Verification items for the finished model (mm, model axes). A direction names the side the tool comes from. Coordinates: 2 decimals unless noted, no trailing zeros. Loops run counter-clockwise (first coordinate to the right, second up) from the corner with the lowest first, then second, coordinate; pieces in that order, holes last. Notation, with made-up numbers: (80.25, 10) - (86.25, 10) arc R28 ccw to (86.25, 44) - close; hole circle Ø8 at (-3, -27). An arc over 180 degrees is marked (long way). Answer as CSV lines item,"result". Start each with the question number.
1. Material ranges on line 1 (X direction, y = -1.5, z = 14); line 2 (Z direction, x = 40.8, y = -11.3); line 3 (Y direction, x = 81.6, z = 13.5), recorded low to high. Write a range as [from, to].
2. Cross-section at D-D (z = 26). Enter the section's corners in (x, y), plus the area to 3 significant figures.
3. Set-up check for faces 1 (the cylindrical face through (70.21, 3.78, 34.17)), 2 (the flat face through (74.84, 6.99, 34.17)), 3 (the flat face through (21.503, 15.216, 5.677)), 4 (the cylindrical face through (60.177, 15.018, 0.143)), 5 (the cylindrical face through (39.759, -11.392, 27.932)): record each of +Z, -Z, +X, -X, +Y, -Y from which the full face is reachable in a straight line by a thin tool's end or side.
4. Cross-section at A-A (z = 20). Enter the section's corners in (x, y).
5. Gauge pin test, flat ends, axial feed: P1, Ø5, axis at x = 35.3, y = 17.5, coming from the +Z side; P2, Ø14.5, axis at x = 40.8, z = 45, coming from the +Y side; P3, Ø4, axis at y = -3.5, z = 41, coming from the +X side. Record the tip position at first contact, or that the pin passes through.
6. Release check for a two-part mould opening along Z. For faces 6 (the cylindrical face through (-7.493, 0.33, 28.594)), 7 (the cylindrical face through (21.423, 15.018, 0.143)), 8 (the cylindrical face through (39.759, -11.392, 52.932)) record: pulls with the +Z half, pulls with the -Z half, needs draft (parallel to the pull), parting line crosses it, or undercut.
7. Cross-section at B-B (x = 39). State how many separate pieces and enclosed holes the cut face has, plus the area to 3 significant figures.
8. Cross-section at C-C (z = 33). Enter the section's corners in (x, y), plus the area to 3 significant figures.
```python
from build123d import *

# Parameters (mm, degrees)
CYLINDER010_R          = 3.2
CYLINDER010_DEPTH      = 40
CYLINDER011_R          = 3.2
CYLINDER011_DEPTH      = 40
CYLINDER012_R          = 8
CYLINDER012_DEPTH      = 1.2
CYLINDER013_R          = 8
CYLINDER013_DEPTH      = 1.2
BOX002_W               = 2
BOX002_H               = 10
BOX002_DEPTH           = 60
BOX002_PLACEMENT_ANGLE = 45
BOX003_W               = 2
BOX003_H               = 10
BOX003_DEPTH           = 60
BOX003_PLACEMENT_ANGLE = 45
CYLINDER006_R          = 2
CYLINDER006_DEPTH      = 20
CYLINDER007_R          = 2
CYLINDER007_DEPTH      = 20
CYLINDER008_R          = 2
CYLINDER008_DEPTH      = 20
CYLINDER009_R          = 2
CYLINDER009_DEPTH      = 20
CYLINDER005_R          = 12
CYLINDER005_DEPTH      = 4
CYLINDER004_R          = 5.5
CYLINDER004_DEPTH      = 20
CYLINDER002_R          = 7.5
CYLINDER002_DEPTH      = 58
CYLINDER_R             = 7.5
CYLINDER_DEPTH         = 58
BOX001_W               = 81.6
BOX001_H               = 33
BOX001_DEPTH           = 11
CHAMFER_1_SIZE2        = 35
CHAMFER_1_SIZE         = 15
CHAMFER_2_SIZE2        = 35
CHAMFER_2_SIZE         = 15
CYLINDER001_R          = 12
CYLINDER001_DEPTH      = 58
CYLINDER003_R          = 12
CYLINDER003_DEPTH      = 58
BOX_W                  = 81.6
BOX_H                  = 12
BOX_DEPTH              = 58
FILLET_R               = 0.5


with BuildPart() as cylinder:
    # Cylinder010 → Cylinder010 (new body)
    with BuildSketch(Plane(origin=(40.8, 20, 20), x_dir=(1, 0, 0), z_dir=(0, -1, 0))):
        Circle(CYLINDER010_R)
    extrude(amount=CYLINDER010_DEPTH)


with BuildPart() as cylinder001:
    # Cylinder011 → Cylinder011 (new body)
    with BuildSketch(Plane(origin=(40.8, 20, 45), x_dir=(1, 0, 0), z_dir=(0, -1, 0))):
        Circle(CYLINDER011_R)
    extrude(amount=CYLINDER011_DEPTH)


with BuildPart() as cylinder002:
    # Cylinder012 → Cylinder012 (new body)
    with BuildSketch(Plane(origin=(40.8, -10.8, 20), x_dir=(1, 0, 0), z_dir=(0, -1, 0))):
        Circle(CYLINDER012_R)
    extrude(amount=CYLINDER012_DEPTH)


with BuildPart() as cylinder003:
    # Cylinder013 → Cylinder013 (new body)
    with BuildSketch(Plane(origin=(40.8, -10.8, 45), x_dir=(1, 0, 0), z_dir=(0, -1, 0))):
        Circle(CYLINDER013_R)
    extrude(amount=CYLINDER013_DEPTH)


with BuildPart() as obj1:
    # Box002 → Box002 (new body)
    with BuildSketch(Plane.XY):
        with Locations((1, 5)):
            Rectangle(BOX002_W, BOX002_H)
    extrude(amount=BOX002_DEPTH)


with BuildPart() as obj1_1:
    # Box002 placement: moved
    add(obj1.part.moved(Location((77, 2, 11))).rotate(Axis((77, 2, 11), (0, 0, 1)), BOX002_PLACEMENT_ANGLE))


with BuildPart() as obj2:
    # Box003 → Box003 (new body)
    with BuildSketch(Plane.XY):
        with Locations((1, 5)):
            Rectangle(BOX003_W, BOX003_H)
    extrude(amount=BOX003_DEPTH)


with BuildPart() as obj2_1:
    # Box003 placement: moved
    add(obj2.part.moved(Location((3, 3, 11))).rotate(Axis((3, 3, 11), (0, 0, -1)), BOX003_PLACEMENT_ANGLE))


with BuildPart() as zylinder006:
    # Cylinder006 → Cylinder006 (new body)
    with BuildSketch(Plane(origin=(35.3, 6.5, 0), x_dir=(1, 0, 0), z_dir=(0, 0, 1))):
        Circle(CYLINDER006_R)
    extrude(amount=CYLINDER006_DEPTH)


with BuildPart() as zylinder007:
    # Cylinder007 → Cylinder007 (new body)
    with BuildSketch(Plane(origin=(35.3, 17.5, 0), x_dir=(1, 0, 0), z_dir=(0, 0, 1))):
        Circle(CYLINDER007_R)
    extrude(amount=CYLINDER007_DEPTH)


with BuildPart() as zylinder008:
    # Cylinder008 → Cylinder008 (new body)
    with BuildSketch(Plane(origin=(46.3, 6.5, 0), x_dir=(1, 0, 0), z_dir=(0, 0, 1))):
        Circle(CYLINDER008_R)
    extrude(amount=CYLINDER008_DEPTH)


with BuildPart() as zylinder009:
    # Cylinder009 → Cylinder009 (new body)
    with BuildSketch(Plane(origin=(46.3, 17.5, 0), x_dir=(1, 0, 0), z_dir=(0, 0, 1))):
        Circle(CYLINDER009_R)
    extrude(amount=CYLINDER009_DEPTH)


with BuildPart() as zylinder005:
    # Cylinder005 → Cylinder005 (new body)
    with BuildSketch(Plane(origin=(40.8, 12, 7), x_dir=(1, 0, 0), z_dir=(0, 0, 1))):
        Circle(CYLINDER005_R)
    extrude(amount=CYLINDER005_DEPTH)


with BuildPart() as zylinder004:
    # Cylinder004 → Cylinder004 (new body)
    with BuildSketch(Plane(origin=(40.8, 12, 0), x_dir=(1, 0, 0), z_dir=(0, 0, 1))):
        Circle(CYLINDER004_R)
    extrude(amount=CYLINDER004_DEPTH)


with BuildPart() as zylinder002:
    # Cylinder002 → Cylinder002 (new body)
    with BuildSketch(Plane(origin=(81.6, 0, 0), x_dir=(1, 0, 0), z_dir=(0, 0, 1))):
        Circle(CYLINDER002_R)
    extrude(amount=CYLINDER002_DEPTH)


with BuildPart() as zylinder:
    # Cylinder → Cylinder (new body)
    with BuildSketch(Plane.XY):
        Circle(CYLINDER_R)
    extrude(amount=CYLINDER_DEPTH)


with BuildPart() as chamfer_body:
    # Box001 → Box001 (new body)
    with BuildSketch(Plane(origin=(0, -12, 0), x_dir=(1, 0, 0), z_dir=(0, 0, 1))):
        with Locations((40.8, 16.5)):
            Rectangle(BOX001_W, BOX001_H)
    extrude(amount=BOX001_DEPTH)

    # Chamfer 1
    chamfer_1_edges = [chamfer_body.edges().sort_by_distance(p)[0] for p in [
        (81.6, 21, 5.5),
    ]]
    chamfer_1_side = chamfer_body.faces().sort_by_distance((81.6, 4.5, 5.5))[0]
    chamfer(chamfer_1_edges, length=CHAMFER_1_SIZE, length2=CHAMFER_1_SIZE2, reference=chamfer_1_side)

    # Chamfer 2
    chamfer_2_edges = [chamfer_body.edges().sort_by_distance(p)[0] for p in [
        (0, 21, 5.5),
    ]]
    chamfer_2_side = chamfer_body.faces().sort_by_distance((0, 4.5, 5.5))[0]
    chamfer(chamfer_2_edges, length=CHAMFER_2_SIZE, length2=CHAMFER_2_SIZE2, reference=chamfer_2_side)


with BuildPart() as zylinder001:
    # Cylinder001 → Cylinder001 (new body)
    with BuildSketch(Plane.XY):
        Circle(CYLINDER001_R)
    extrude(amount=CYLINDER001_DEPTH)


with BuildPart() as zylinder003:
    # Cylinder003 → Cylinder003 (new body)
    with BuildSketch(Plane(origin=(81.6, 0, 0), x_dir=(1, 0, 0), z_dir=(0, 0, 1))):
        Circle(CYLINDER003_R)
    extrude(amount=CYLINDER003_DEPTH)


with BuildPart() as fillet_body:
    # Box → Box (new body)
    with BuildSketch(Plane(origin=(0, -12, 0), x_dir=(1, 0, 0), z_dir=(0, 0, 1))):
        with Locations((40.8, 6)):
            Rectangle(BOX_W, BOX_H)
    extrude(amount=BOX_DEPTH)

    # Fusion: union Chamfer body, Zylinder001, Zylinder003
    add(chamfer_body.part)
    add(zylinder001.part)
    add(zylinder003.part)

    # Cut: cut Zylinder
    add(zylinder.part, mode=Mode.SUBTRACT)

    # Cut001: cut Zylinder002
    add(zylinder002.part, mode=Mode.SUBTRACT)

    # Cut002: cut Zylinder004
    add(zylinder004.part, mode=Mode.SUBTRACT)

    # Cut003: cut Zylinder005
    add(zylinder005.part, mode=Mode.SUBTRACT)

    # Cut004: cut Zylinder009
    add(zylinder009.part, mode=Mode.SUBTRACT)

    # Cut005: cut Zylinder008
    add(zylinder008.part, mode=Mode.SUBTRACT)

    # Cut006: cut Zylinder007
    add(zylinder007.part, mode=Mode.SUBTRACT)

    # Cut007: cut Zylinder006
    add(zylinder006.part, mode=Mode.SUBTRACT)

    # Cut008: cut obj2
    add(obj2_1.part, mode=Mode.SUBTRACT)

    # Cut009: cut obj1
    add(obj1_1.part, mode=Mode.SUBTRACT)

    # Cut010: cut Cylinder003
    add(cylinder003.part, mode=Mode.SUBTRACT)

    # Cut011: cut Cylinder002
    add(cylinder002.part, mode=Mode.SUBTRACT)

    # Cut012: cut Cylinder001
    add(cylinder001.part, mode=Mode.SUBTRACT)

    # Cut013: cut Cylinder
    add(cylinder.part, mode=Mode.SUBTRACT)

    # Fillet
    fillet_edges = [fillet_body.edges().sort_by_distance(p)[0] for p in [
        (-11.296167, 4.049272, 0),
        (40.8, -12, 0),
        (21.311771, 15.133616, 0),
        (40.8, 21, 0),
        (60.288229, 15.133616, 0),
        (86.724329, 10.850864, 0),
        (90.085281, -8.485281, 0),
    ]]
    fillet(fillet_edges, radius=FILLET_R)


solid = fillet_body.part
```
Values follow:
1,line 1,"x = [-11.91, -7.35], [7.35, 74.25], [88.95, 93.51]"
1,line 2,"z = [0, 12], [28, 37], [53, 58]"
1,line 3,"y = [-12, -7.5], [7.5, 12]"
2,outline,"(0, -12) - (35.51, -12) - (35.51, -10.8) - (46.09, -10.8) - (46.09, -12) - (81.6, -12) arc R12 ccw (long way) to (73.23, 8.6) - (76.41, 5.42) arc R7.5 cw (long way) to (75.16, 3.84) - (71.91, 7.09) arc R12 ccw to (69.6, 0) - (12, 0) arc R12 ccw to (9.78, 6.95) - (6.53, 3.7) arc R7.5 cw (long way) to (5.3, 5.3) - (8.49, 8.49) arc R12 ccw (long way) to start"
2,area,"1,270 mm²"
3,face 1,"+Z, +Y"
3,face 2,"+Z"
3,face 3,"+Z, -Z, +Y"
3,face 4,"-Z, +Y"
3,face 5,"-Y"
4,outline,"(0, -12) - (32.8, -12) - (32.8, -10.8) - (37.6, -10.8) - (37.6, 0) - (12, 0) arc R12 ccw to (9.78, 6.95) - (6.53, 3.7) arc R7.5 cw (long way) to (5.3, 5.3) - (8.49, 8.49) arc R12 ccw (long way) to start; (44, -10.8) - (48.8, -10.8) - (48.8, -12) - (81.6, -12) arc R12 ccw (long way) to (73.23, 8.6) - (76.41, 5.42) arc R7.5 cw (long way) to (75.16, 3.84) - (71.91, 7.09) arc R12 ccw to (69.6, 0) - (44, 0) - close"
5,P1,"stops at z = 7"
5,P2,"stops at y = 0"
5,P3,"stops at x = 93.51"
6,face 6,"needs draft"
6,face 7,"pulls with the -Z half"
6,face 8,"undercut"
7,separate pieces,"4"
7,enclosed holes,"0"
7,area,"619 mm²"
8,outline,"(0, -12) - (81.6, -12) arc R12 ccw (long way) to (73.23, 8.6) - (76.41, 5.42) arc R7.5 cw (long way) to (75.16, 3.84) - (71.91, 7.09) arc R12 ccw to (69.6, 0) - (12, 0) arc R12 ccw to (9.78, 6.95) - (6.53, 3.7) arc R7.5 cw (long way) to (5.3, 5.3) - (8.49, 8.49) arc R12 ccw (long way) to start"
8,area,"1,290 mm²"
